```python
from build123d import *

# Parameters (mm, degrees)
F1_DEPTH  = 247.3
F3_DEPTH  = 300
F4_DEPTH  = 50
F5_DEPTH  = 59.1
F6_DEPTH  = 300
F7_DEPTH  = 300
F8_DEPTH  = 17.109
F9_DEPTH  = 1.9
F10_DEPTH = 1
F11_DEPTH = 3


with BuildPart() as f1:
    # F0 (on Front) → F1 (new body)
    with BuildSketch(Plane.XZ):
        Polygon((-78.8866152354, 43.4383174348), (-78.6296018241, 42.9628188217), (-78.6296018241, 102.819841868), (-127.7663317061, 102.819841868), (-96.9769939736, 76.9071934711), align=None)
        Polygon((-79.7663317061, 42.9628188217), (-97.7663317061, 76.264485822), (-127.7663317061, 101.5128188217), (-157.7663317061, 76.264485822), (-175.7663317061, 42.9628188217), align=None)
        Polygon((-127.7663317061, 101.5128188217), (-97.7663317061, 76.264485822), (-79.7663317061, 42.9628188217), (-78.6296018241, 42.9628188217), (-78.8866152354, 43.4383174348), (-96.9769939736, 76.9071934711), (-127.7663317061, 102.819841868), (-158.5556694386, 76.9071934711), (-176.9030615881, 42.9628188217), (-175.7663317061, 42.9628188217), (-157.7663317061, 76.264485822), align=None)
        Polygon((-176.9030615881, 102.819841868), (-176.9030615881, 42.9628188217), (-158.5556694386, 76.9071934711), (-127.7663317061, 102.819841868), align=None)
    extrude(amount=-F1_DEPTH)

    # F0 (on Front) → F3 (cut)
    with BuildSketch(Plane.XZ):
        Polygon((-78.8866152354, 43.4383174348), (-78.6296018241, 42.9628188217), (-78.6296018241, 102.819841868), (-127.7663317061, 102.819841868), (-96.9769939736, 76.9071934711), align=None)
    extrude(amount=-F3_DEPTH, mode=Mode.SUBTRACT)

    # F2 (on face) → F4 (join)
    with BuildSketch(Plane.YZ.offset(-78.6296018241)):
        Polygon((142.2357864376, 84.2340554304), (123.65, 102.819841868), (123.65, 101.4056283057), (141.5286796564, 83.5269486492), align=None)
        Polygon((123.65, 101.4056283057), (123.65, 102.819841868), (105.0642135624, 84.2340554304), (105.7713203436, 83.5269486492), align=None)
    extrude(amount=-F4_DEPTH)

    # F2 (on face) → F5 (join)
    with BuildSketch(Plane.YZ.offset(-78.6296018241)):
        Polygon((103.65, 42.9628188217), (123.65, 42.9628188217), (123.65, 82.819841868), (106.4784271247, 82.819841868), (105.0642135624, 82.819841868), (103.65, 82.819841868), align=None)
        Polygon((123.65, 42.9628188217), (143.65, 42.9628188217), (143.65, 82.819841868), (142.2357864376, 82.819841868), (140.8215728753, 82.819841868), (123.65, 82.819841868), align=None)
    extrude(amount=-F5_DEPTH)

    # F2 (on face) → F6 (cut)
    with BuildSketch(Plane.YZ.offset(-78.6296018241)):
        Polygon((247.3, 42.9628188217), (247.3, 102.819841868), (123.65, 102.819841868), (142.2357864376, 84.2340554304), (141.5286796564, 83.5269486492), (142.2357864376, 82.819841868), (143.65, 82.819841868), (143.65, 42.9628188217), align=None)
        Polygon((105.0642135624, 84.2340554304), (123.65, 102.819841868), (0, 102.819841868), (0, 42.9628188217), (103.65, 42.9628188217), (103.65, 82.819841868), (105.0642135624, 82.819841868), (105.7713203436, 83.5269486492), align=None)
        Polygon((123.65, 42.9628188217), (143.65, 42.9628188217), (143.65, 82.819841868), (142.2357864376, 82.819841868), (140.8215728753, 82.819841868), (123.65, 82.819841868), align=None)
        Polygon((103.65, 42.9628188217), (123.65, 42.9628188217), (123.65, 82.819841868), (106.4784271247, 82.819841868), (105.0642135624, 82.819841868), (103.65, 82.819841868), align=None)
    extrude(amount=-F6_DEPTH, mode=Mode.SUBTRACT)

    # F0 (on Front) → F7 (cut)
    with BuildSketch(Plane.XZ):
        Polygon((-176.9030615881, 102.819841868), (-176.9030615881, 42.9628188217), (-158.5556694386, 76.9071934711), (-127.7663317061, 102.819841868), align=None)
        Polygon((-127.7663317061, 101.5128188217), (-97.7663317061, 76.264485822), (-79.7663317061, 42.9628188217), (-78.6296018241, 42.9628188217), (-78.8866152354, 43.4383174348), (-96.9769939736, 76.9071934711), (-127.7663317061, 102.819841868), (-158.5556694386, 76.9071934711), (-176.9030615881, 42.9628188217), (-175.7663317061, 42.9628188217), (-157.7663317061, 76.264485822), align=None)
        Polygon((-79.7663317061, 42.9628188217), (-97.7663317061, 76.264485822), (-127.7663317061, 101.5128188217), (-157.7663317061, 76.264485822), (-175.7663317061, 42.9628188217), align=None)
    extrude(amount=-F7_DEPTH, mode=Mode.SUBTRACT)

    # F2 (on face) → F8 (join)
    with BuildSketch(Plane.YZ.offset(-78.6296018241)):
        Polygon((123.65, 101.4056283057), (123.65, 102.819841868), (105.0642135624, 84.2340554304), (105.7713203436, 83.5269486492), align=None)
        Polygon((142.2357864376, 84.2340554304), (123.65, 102.819841868), (123.65, 101.4056283057), (141.5286796564, 83.5269486492), align=None)
    extrude(amount=F8_DEPTH)

    # F9 (add): a face of the model
    f9_faces = [f1.faces().sort_by_distance(p)[0] for p in [
        (-61.5206018241, 114.6532437055, 93.2308117249),
    ]]
    extrude(f9_faces, amount=F9_DEPTH)

    # F10 (add): a face of the model
    f10_faces = [f1.faces().sort_by_distance(p)[0] for p in [
        (-59.6206018241, 114.6532437055, 93.2308117249),
    ]]
    extrude(f10_faces, amount=F10_DEPTH)

    # F11 (add): a face of the model
    f11_faces = [f1.faces().sort_by_distance(p)[0] for p in [
        (-58.6206018241, 114.6532437055, 93.2308117249),
    ]]
    extrude(f11_faces, amount=F11_DEPTH)


solid = f1.part
```
For this review, take the finished solid that the model builds, in its own axes (mm). A direction names the side the tool comes from. Round coordinates to 2 decimals unless told otherwise and drop trailing zeros. Loops run counter-clockwise (first coordinate to the right, second up) from the corner with the lowest first, then second, coordinate; pieces in that order, holes last.
Q1. Machinability: for faces 1 (the face through (-84.18, 114.49, 93.66)), 2 (the face through (-83.517, 114.586, 92.341)), which of the approach directions +Z, -Z, +X, -X, +Y, -Y give a long, thin tool a straight path to every point of the face, cutting with its end or side? Answer none if there is none.
Result sheet:
face 1: +Z, +X, -X, -Y
face 2: -Z, +X, -X
Q2. Add section B-B on x = -75. Write out the cut boundary in (y, z), plus the area to 3 significant figures.
Result sheet:
outline: (105.06, 84.23) - (105.77, 83.53) - (123.65, 101.41) - (141.53, 83.53) - (142.24, 84.23) - (123.65, 102.82) - close
area: 51.6 mm2
Q3. Insertion check: pin 1 Ø5 at (y, z) = (129, 91.5) entering from +X; pin 2 Ø1.5 at (x, z) = (-77.5, 87.5) entering from -Y; pin 3 Ø8 at (x, z) = (-107, 90.5) entering from +Y; pin 4 Ø6 at (x, z) = (-82.5, 91) entering from -Y. Each pin has a flat end and moves straight along its axis. Give the tip position at first contact, or say it passes through.
Result sheet:
pin 1: passes through
pin 2: stops at y = 107.58
pin 3: stops at y = 139.97
pin 4: stops at y = 108.83
Q4. Mouldability with a two-part tool opening along Y and no side actions: class faces 3 (the face through (-55.621, 119.4, 97.5)), 4 (the face through (-84.18, 133.07, 93.4)), 5 (the face through (-83.517, 132.464, 92.591)) as +Y half, -Y half, draft (parallel to the pull), parting line (faces both ways), or undercut.
Result sheet:
face 3: draft
face 4: +Y half
face 5: undercut
Q5. Add section C-C on z = 87. Write out the cut boundary in (x, y).
Result sheet:
outline: (-108.97, 107.83) - (-55.62, 107.83) - (-55.62, 109.24) - (-108.97, 109.24) - close; (-108.97, 138.06) - (-55.62, 138.06) - (-55.62, 139.47) - (-108.97, 139.47) - close
Q6. Add section A-A on z = 91. Write out the cut boundary in (x, y).
Result sheet:
outline: (-113.72, 111.83) - (-55.62, 111.83) - (-55.62, 113.24) - (-113.72, 113.24) - close; (-113.72, 134.06) - (-55.62, 134.06) - (-55.62, 135.47) - (-113.72, 135.47) - close
Q7. To check wall thickness, follow line 1 along Y through (x, z) = (-63, 100.75); line 2 along Y through (x, z) = (-60, 95.5); line 3 along Z through (x, y) = (-123, 124). State the ranges of each line that lie inside material, in increasing order.
Result sheet:
line 1: y = 121.58 to 122.99, 124.31 to 125.72
line 2: y = 116.33 to 117.74, 129.56 to 130.97
line 3: z = 101.06 to 102.47
Q8. Add section D-D on y = 138.5. Write out the cut boundary in (x, z).
Result sheet:
outline: (-110.12, 87.97) - (-108.44, 86.56) - (-55.62, 86.56) - (-55.62, 87.97) - close
